Source: CAD feature listing. Evaluate the final solid. Frame: model axes, mm. A direction names the side the tool comes from. Give positions to 0.01 mm unless a question says otherwise; leave off trailing zeros. Loops run counter-clockwise (first coordinate to the right, second up) from the corner with the lowest first, then second, coordinate; pieces in that order, holes last.
```python
from build123d import *

# Parameters (mm, degrees)
EXTRUDE_1_DEPTH      = 3
EXTRUDE_1_DEPTH_BACK = 3
SKETCH_1_4_R         = 12
SKETCH_1_4_R_2       = 4.1
EXTRUDE_2_DEPTH      = 4.5


with BuildPart() as part:
    # 草图1 → 凸台-拉伸1 (new, two sides: drawn at the far end of the back side and taken through both)
    with BuildSketch(Plane.XY.offset(-EXTRUDE_1_DEPTH_BACK)):
        with BuildLine():
            Line((42.062746067, 9), (-42.062746067, 9))
            ThreePointArc((-42.062746067, 9), (-39.062746067, 4.937253933), (-38, 0))
            ThreePointArc((-38, 0), (-39.062746067, -4.937253933), (-42.062746067, -9))
            Line((-42.062746067, -9), (42.062746067, -9))
            ThreePointArc((42.062746067, -9), (38, 0), (42.062746067, 9))
        make_face()
    extrude(amount=EXTRUDE_1_DEPTH + EXTRUDE_1_DEPTH_BACK)

    # 草图1<4> → 凸台-拉伸2 (add, symmetric)
    # profile 1 of 2: a face of its own
    with BuildSketch(Plane.XY):
        with Locations((-50, 0)):
            Circle(SKETCH_1_4_R)
        with Locations((-50, 0)):
            Circle(SKETCH_1_4_R_2, mode=Mode.SUBTRACT)
    # profile 2 of 2: a face of its own
    with BuildSketch(Plane.XY):
        with Locations((50, 0)):
            Circle(SKETCH_1_4_R)
        with Locations((50, 0)):
            Circle(SKETCH_1_4_R_2, mode=Mode.SUBTRACT)
    extrude(amount=EXTRUDE_2_DEPTH, both=True)


solid = part.part
```
(1) Section D-D, the plane y = 10.75. Return the cut outline in (x, z), then the cut area to 3 significant figures.
A:
outline: (-55.33, -4.5) - (-44.67, -4.5) - (-44.67, 4.5) - (-55.33, 4.5) - close; (44.67, -4.5) - (55.33, -4.5) - (55.33, 4.5) - (44.67, 4.5) - close
area: 192 mm2
(2) Section B-B, the plane y = 0. Return the cut outline in (x, z).
A:
outline: (-62, -4.5) - (-54.1, -4.5) - (-54.1, 4.5) - (-62, 4.5) - close; (-45.9, -4.5) - (-38, -4.5) - (-38, -3) - (38, -3) - (38, -4.5) - (45.9, -4.5) - (45.9, 4.5) - (38, 4.5) - (38, 3) - (-38, 3) - (-38, 4.5) - (-45.9, 4.5) - close; (54.1, -4.5) - (62, -4.5) - (62, 4.5) - (54.1, 4.5) - close
(3) Reachability of faces 1 (the cylindrical face through (45.904, 0.18, -0.063)), 2 (the flat face through (1, 9, 0)), 3 (the flat face through (-1, -9, 0)) from +Z, -Z, +X, -X, +Y, -Y: full face, straight path, thin tool, end or side. Return the list, or none.
A:
face 1: +Z, -Z
face 2: +Z, -Z, +Y
face 3: +Z, -Z, -Y
(4) First-contact query: pin 1 (5 mm diameter, centred on x = -10, z = 0, fed in from +Y); pin 2 (3 mm diameter, centred on x = 4.5, z = 2.5, fed in from -Y); pin 3 (1 mm diameter, centred on x = 24, y = -4.5, fed in from +Z); pin 4 (7.5 mm diameter, centred on x = 50, y = 0, fed in from +Z). Flat tips, straight axial feed; report the tip coordinate or a pass-through.
A:
pin 1: stops at y = 9
pin 2: stops at y = -9
pin 3: stops at z = 3
pin 4: passes through
(5) Ray query, line 1 along Y through (x, z) = (-50, -2.75); line 2 along X through (y, z) = (-2.25, 3.5); line 3 along Z through (x, y) = (17, -4.75). Return the intervals inside material, ascending.
A:
line 1: y = -12 to -4.1, 4.1 to 12
line 2: x = -61.79 to -53.43, -46.57 to -38.21, 38.21 to 46.57, 53.43 to 61.79
line 3: z = -3 to 3
(6) Mould query, pull axis X, two halves, no side actions, for faces 4 (the flat face through (-1, 0, -3)), 5 (the flat face through (-45, 0, -4.5)). Classes: pulls with the +X half, pulls with the -X half, needs draft (parallel to the pull), parting line crosses it, or undercut.
A:
face 4: undercut
face 5: needs draft
(7) Section A-A, the plane x = 50. Return the cut outline in (y, z), then the cut area to 3 significant figures.
A:
outline: (-12, -4.5) - (-4.1, -4.5) - (-4.1, 4.5) - (-12, 4.5) - close; (4.1, -4.5) - (12, -4.5) - (12, 4.5) - (4.1, 4.5) - close
area: 142 mm2
(8) Section C-C, the plane z = -1.5. Return the cut outline in (x, y), then the cut area to 3 significant figures.
A:
outline: (-42.06, -9) - (42.06, -9) arc R12 ccw (long way) to (42.06, 9) - (-42.06, 9) arc R12 ccw (long way) to start; hole circle Ø8.2 at (-50, 0); hole circle Ø8.2 at (50, 0)
area: 2,210 mm2
